from build123d import *

# Parameters (mm, degrees)
SKETCH1_W           = 70
SKETCH1_H           = 70
BOSS_EXTRUDE1_DEPTH = 1
SKETCH3_W           = 11
SKETCH3_H           = 11
BOSS_EXTRUDE2_DEPTH = 0.2
SKETCH4_W           = 5.900984105
SKETCH4_H           = 4.163778505
CUT_EXTRUDE3_DEPTH  = 0.2


with BuildPart() as part:
    # Sketch1 → Boss-Extrude1 (new body)
    with BuildSketch(Plane.XY):
        with Locations((-31.007117438, 12.099644128)):
            Rectangle(SKETCH1_W, SKETCH1_H)
    extrude(amount=BOSS_EXTRUDE1_DEPTH)

    # Sketch3 → Boss-Extrude2 (add)
    with BuildSketch(Plane.XY.offset(1)):
        Polygon((-48.757117438, 42.099644128), (-50.007117438, 42.099644128), (-50.007117438, 31.099644128), (-61.007117438, 31.099644128), (-61.007117438, 29.849644128), (-50.007117438, 29.849644128), (-50.007117438, 18.849644128), (-61.007117438, 18.849644128), (-61.007117438, 17.599644128), (-50.007117438, 17.599644128), (-50.007117438, 6.599644128), (-61.007117438, 6.599644128), (-61.007117438, 5.349644128), (-50.007117438, 5.349644128), (-50.007117438, -5.650355872), (-61.007117438, -5.650355872), (-61.007117438, -6.900355872), (-50.007117438, -6.900355872), (-50.007117438, -17.900355872), (-48.757117438, -17.900355872), (-48.757117438, -6.900355872), (-37.757117438, -6.900355872), (-37.757117438, -17.900355872), (-36.507117438, -17.900355872), (-36.507117438, -6.900355872), (-25.507117438, -6.900355872), (-25.507117438, -17.900355872), (-24.257117438, -17.900355872), (-24.257117438, -6.900355872), (-13.257117438, -6.900355872), (-13.257117438, -17.900355872), (-12.007117438, -17.900355872), (-12.007117438, -6.900355872), (-1.007117438, -6.900355872), (-1.007117438, -5.650355872), (-12.007117438, -5.650355872), (-12.007117438, 5.349644128), (-1.007117438, 5.349644128), (-1.007117438, 6.599644128), (-12.007117438, 6.599644128), (-12.007117438, 17.599644128), (-1.007117438, 17.599644128), (-1.007117438, 18.849644128), (-12.007117438, 18.849644128), (-12.007117438, 29.849644128), (-1.007117438, 29.849644128), (-1.007117438, 31.099644128), (-12.007117438, 31.099644128), (-12.007117438, 42.099644128), (-13.257117438, 42.099644128), (-13.257117438, 31.099644128), (-24.257117438, 31.099644128), (-24.257117438, 42.099644128), (-25.507117438, 42.099644128), (-25.507117438, 31.099644128), (-36.507117438, 31.099644128), (-36.507117438, 42.099644128), (-37.757117438, 42.099644128), (-37.757117438, 31.099644128), (-48.757117438, 31.099644128), align=None)
        with Locations((-43.257117438, -0.150355872)):
            Rectangle(SKETCH3_W, SKETCH3_H, mode=Mode.SUBTRACT)
        with Locations((-31.007117438, -0.150355872)):
            Rectangle(SKETCH3_W, SKETCH3_H, mode=Mode.SUBTRACT)
        with Locations((-18.757117438, -0.150355872)):
            Rectangle(SKETCH3_W, SKETCH3_H, mode=Mode.SUBTRACT)
        with Locations((-43.257117438, 12.099644128)):
            Rectangle(SKETCH3_W, SKETCH3_H, mode=Mode.SUBTRACT)
        with Locations((-43.257117438, 24.349644128)):
            Rectangle(SKETCH3_W, SKETCH3_H, mode=Mode.SUBTRACT)
        with Locations((-31.007117438, 12.099644128)):
            Rectangle(SKETCH3_W, SKETCH3_H, mode=Mode.SUBTRACT)
        with Locations((-18.757117438, 12.099644128)):
            Rectangle(SKETCH3_W, SKETCH3_H, mode=Mode.SUBTRACT)
        with Locations((-31.007117438, 24.349644128)):
            Rectangle(SKETCH3_W, SKETCH3_H, mode=Mode.SUBTRACT)
        with Locations((-18.757117438, 24.349644128)):
            Rectangle(SKETCH3_W, SKETCH3_H, mode=Mode.SUBTRACT)
    extrude(amount=BOSS_EXTRUDE2_DEPTH)

    # Sketch4 → Cut-Extrude3 (cut)
    with BuildSketch(Plane.XY.offset(1.2)):
        with Locations((-50.439270902, -17.397627398)):
            Rectangle(SKETCH4_W, SKETCH4_H)
    extrude(amount=-CUT_EXTRUDE3_DEPTH, mode=Mode.SUBTRACT)


solid = part.part
Input: part model. Units: mm. Frame: model coordinates. A direction names the side the tool comes from. Coordinates: 2 decimals unless noted, no trailing zeros. Order: outer loops, then holes, each group sorted by start corner. A loop starts at its lowest first (then second) coordinate and runs counter-clockwise, first axis right, second up. Notation, with made-up numbers: M 45.25,7 L 58.25,7 A6 cw 58.25,15 Z; hole C -13.75,25.5 d5. An arc over 180 degrees is marked long. Answer as CSV lines item,"result".
1. Access query for faces 3 (the flat face through (-31, 13, 0)), 4 (the flat face through (-31, 12, 1)). Directions: +Z, -Z, +X, -X, +Y, -Y. A direction counts if a zero-diameter tool reaches every point of the face in a straight line with its end or side. Return the directions, or none.
Reported:
face 3,"-Z, +X, -X, +Y, -Y"
face 4,"+Z"
2. Pull-direction query (X, two-part tool) for faces 1 (the flat face through (-55, 13, 1)), 2 (the flat face through (-33, 6, 1.2)); classes: released by +X, released by -X, zero draft, split by the parting line, or undercut.
Reported:
face 1,"undercut"
face 2,"zero draft"
3. First-contact query: P1, Ø3.5, axis at x = -45, y = -0.5, coming from the +Z side. Flat tip, straight axial feed; report the tip coordinate or a pass-through.
Reported:
P1,"z = 1"
4. Section B-B (y = 27.5). Return the cut outline in (x, z).
Reported:
outline,"M -66.01,0 L 3.99,0 L 3.99,1 L -12.01,1 L -12.01,1.2 L -13.26,1.2 L -13.26,1 L -24.26,1 L -24.26,1.2 L -25.51,1.2 L -25.51,1 L -36.51,1 L -36.51,1.2 L -37.76,1.2 L -37.76,1 L -48.76,1 L -48.76,1.2 L -50.01,1.2 L -50.01,1 L -66.01,1 Z"
5. Section A-A (x = -7.5). Return the cut outline in (y, z).
Reported:
outline,"M -22.9,0 L 47.1,0 L 47.1,1 L 31.1,1 L 31.1,1.2 L 29.85,1.2 L 29.85,1 L 18.85,1 L 18.85,1.2 L 17.6,1.2 L 17.6,1 L 6.6,1 L 6.6,1.2 L 5.35,1.2 L 5.35,1 L -5.65,1 L -5.65,1.2 L -6.9,1.2 L -6.9,1 L -22.9,1 Z"
6. Material intervals for line 1 (X direction, y = 38.5, z = 1.1); line 2 (Z direction, x = -48, y = 21.5), sorted ascending. Write a range as from..to.
Reported:
line 1,"-50.01..-48.76, -37.76..-36.51, -25.51..-24.26, -13.26..-12.01"
line 2,"0..1"
